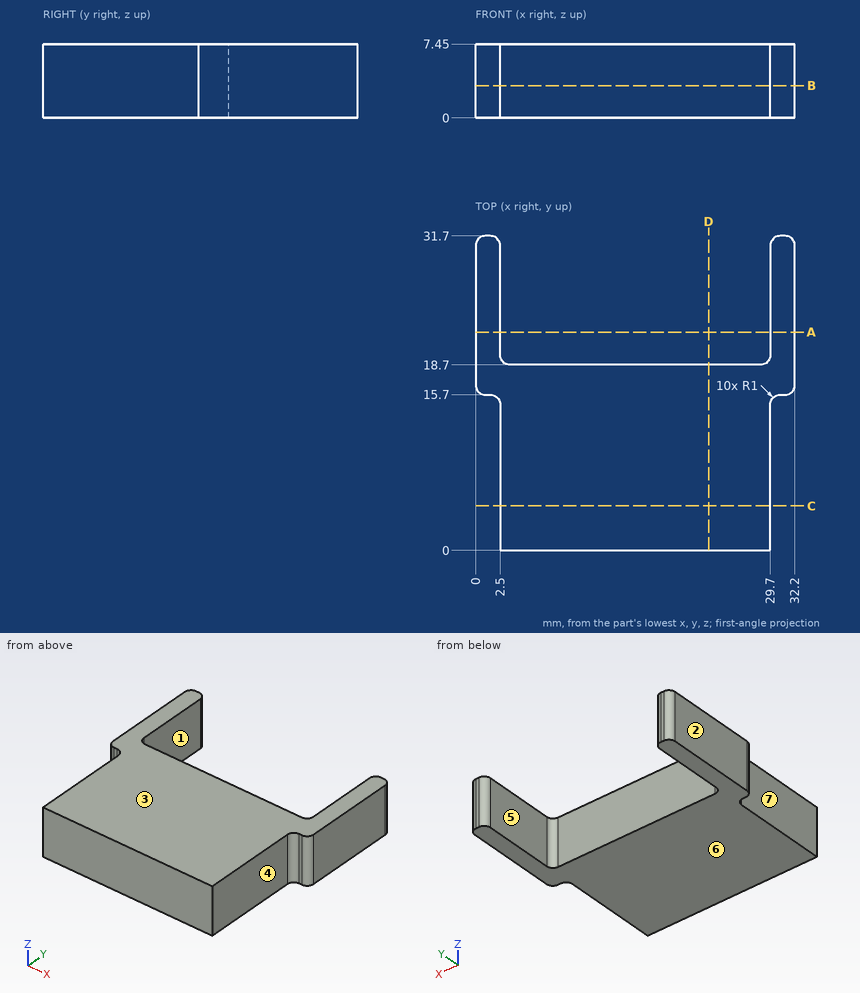
Could you check a few things on this drawing? It's one solid part, dimensions in mm from its lowest x, y, z. A direction names the side the tool comes from. Round coordinates to 2 decimals unless told otherwise and drop trailing zeros. Loops run counter-clockwise (first coordinate to the right, second up) from the corner with the lowest first, then second, coordinate; pieces in that order, holes last.
Q1. I want a section at D-D (x = 23.5). Write out the boundary of the cut face in (y, z), and give its area (3 significant figures).
Q2. Thinking about a two-plate mould opening in X: for the marked faces 1, 2 and 3, which applies, pulls with the +X half, pulls with the -X half, needs draft (parallel to the pull), parting line crosses it, or undercut?
Q3. On a 3-axis mill with a long thin cutter (end or side, diameter ignored), from which of +Z, -Z, +X, -X, +Y, -Y can I reach the whole of each face in a straight line? I mean the marked faces 4, 5, 6 and 7. Say none if no direction works.
Q4. I want a section at A-A (y = 22). Write out the boundary of the cut face in (x, z), and give its area (4 significant figures).
Q5. For P1, Ø2, axis at x = 16, z = 2.5, coming from the +Y side; P2, Ø3.5, axis at y = 7.5, z = 2, coming from the +X side; P3, Ø2, axis at y = 7, z = 5.5, coming from the -X side, each with a flat end and sliding along its axis, tell me the tip position at first contact or that it passes through.
Q6. Please list where these lines run through material, in increasing order: L1, parallel to X at y = 23, z = 2.25; L2, parallel to X at y = 6, z = 1; L3, parallel to Y at x = 23.5, z = 3.25.
Q7. I want a section at C-C (y = 4.5). Write out the boundary of the cut face in (x, z).
Q8. I want a section at B-B (z = 3.25). Write out the boundary of the cut face in (x, y).
Answer below:
1. outline: (0, 0) - (18.7, 0) - (18.7, 7.45) - (0, 7.45) - close
1. area: 139 mm2
2. face 1: undercut
2. face 2: pulls with the -X half
2. face 3: needs draft
3. face 4: +Z, -Z, +X, -Y
3. face 5: +Z, -Z, +Y
3. face 6: -Z, +X, -X, +Y, -Y
3. face 7: +Z, -Z, -X, -Y
4. outline: (0, 0) - (2.5, 0) - (2.5, 7.45) - (0, 7.45) - close; (29.7, 0) - (32.2, 0) - (32.2, 7.45) - (29.7, 7.45) - close
4. area: 37.25 mm2
5. P1: stops at y = 18.7
5. P2: stops at x = 29.7
5. P3: stops at x = 2.5
6. L1: x = 0 to 2.5, 29.7 to 32.2
6. L2: x = 2.5 to 29.7
6. L3: y = 0 to 18.7
7. outline: (2.5, 0) - (29.7, 0) - (29.7, 7.45) - (2.5, 7.45) - close
8. outline: (0, 16.7) arc R1 ccw to (1, 15.7) - (1.5, 15.7) arc R1 cw to (2.5, 14.7) - (2.5, 0) - (29.7, 0) - (29.7, 14.7) arc R1 cw to (30.7, 15.7) - (31.2, 15.7) arc R1 ccw to (32.2, 16.7) - (32.2, 30.7) arc R1 ccw to (31.2, 31.7) - (30.7, 31.7) arc R1 ccw to (29.7, 30.7) - (29.7, 19.7) arc R1 cw to (28.7, 18.7) - (3.5, 18.7) arc R1 cw to (2.5, 19.7) - (2.5, 30.7) arc R1 ccw to (1.5, 31.7) - (1, 31.7) arc R1 ccw to (0, 30.7) - close
